Part print with two shaded views. Sizes in mm from the minimum x, y, z corner. Coordinates: 2 decimals unless noted, no trailing zeros. Loops run counter-clockwise (first coordinate to the right, second up) from the corner with the lowest first, then second, coordinate; pieces in that order, holes last. Notation, with made-up numbers: (89.5, 35.25) -> (103.5, 35.25) arc R31 ccw to (103.5, 68.25) -> close; hole circle Ø7 at (81.25, 75). An arc over 180 degrees is marked (long way). One line per item, written item: value. Start each with the question number.
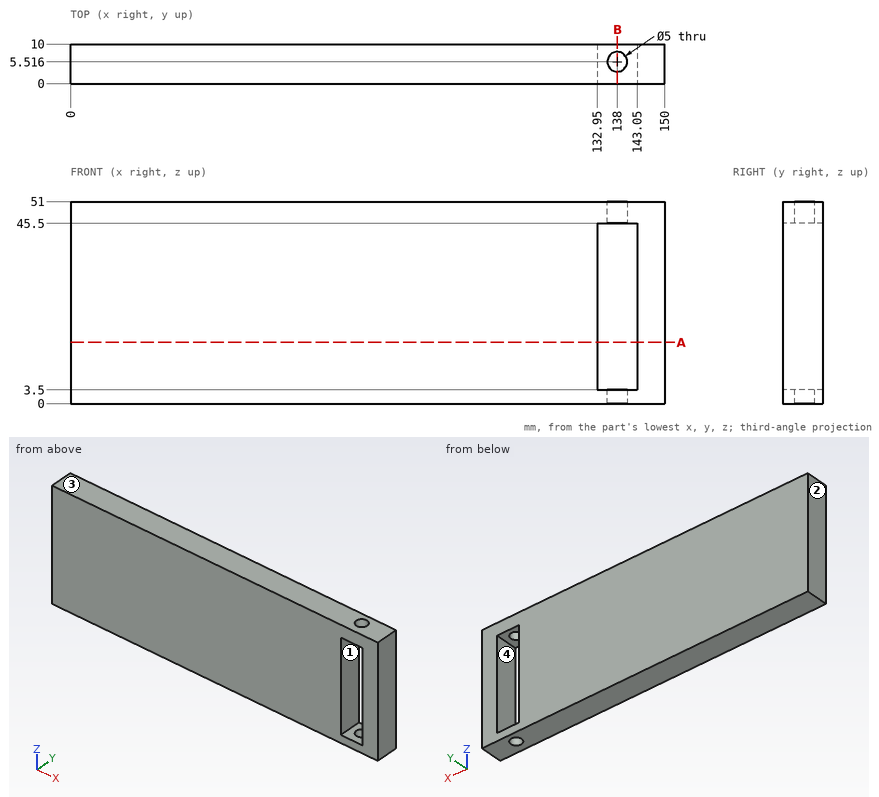
Item 1: Band-saw the part on B-B, the plane x = 138. List the corners of the cut face in (y, z) (1 decimal), and give its area (3 significant figures).
Item 2: Drop a flat-ended pin along its axis: pin 1 Ø4 at (x, y) = (138, 5.52) entering from +Z. Give the stop position or say it passes through.
Item 3: Band-saw the part on A-A, the plane z = 15.5. List the corners of the cut face in (x, y).
Item 4: Probe probe 1 along Y at (x, z) = (138, 49.4) (1 decimal); probe 2 along X at (y, z) = (8, 9.5); probe 3 along Z at (x, y) = (133, 8). List the from-to ranges inside material, lowest first.
Item 5: Two-plate mould, pull along X, no slides. Class the marked faces 1, 2, 3 and 4: +X half, -X half, draft (parallel to the pull), parting line (faces both ways), or undercut.
Worked out:
1. outline: (0, 0) -> (3, 0) -> (3, 3.5) -> (0, 3.5) -> close; (0, 45.5) -> (3, 45.5) -> (3, 51) -> (0, 51) -> close; (8, 0) -> (10, 0) -> (10, 3.5) -> (8, 3.5) -> close; (8, 45.5) -> (10, 45.5) -> (10, 51) -> (8, 51) -> close
1. area: 45.0 mm²
2. pin 1: passes through
3. outline: (0, 0) -> (132.95, 0) -> (132.95, 10) -> (0, 10) -> close; (143.05, 0) -> (150, 0) -> (150, 10) -> (143.05, 10) -> close
4. probe 1: y = 0 to 3, 8 to 10
4. probe 2: x = 0 to 132.95, 143.05 to 150
4. probe 3: z = 0 to 3.5, 45.5 to 51
5. face 1: undercut
5. face 2: -X half
5. face 3: draft
5. face 4: undercut
